```python
from build123d import *

# Parameters (mm, degrees)
F3_DEPTH  = 3
F4_W      = 23
F4_H      = 16
F5_DEPTH  = 11.6
F6_R      = 1.375
F7_DEPTH  = 2.75
F10_R     = 3.5
F11_DEPTH = 1.5
F12_R     = 2
F12_R_2   = 1
F13_DEPTH = 25


with BuildPart() as f1:
    # F0 (on Right) → F1 (revolve)
    with BuildSketch(Plane.YZ):
        Polygon((0, 2), (0, 0), (0.5, 0), (2, 2), align=None)
    revolve(axis=Axis((0, 0, 1), (0, 0, -1)))

    # F2 (on face) → F3 (join)
    with BuildSketch(Plane.XY.offset(2)):
        Polygon((2.020726, 3.5), (-2.020726, 3.5), (-4.041452, 0), (-2.020726, -3.5), (2.020726, -3.5), (4.041452, 0), align=None)
    extrude(amount=F3_DEPTH)

    # F4 (on face) → F5 (join)
    with BuildSketch(Plane.XY.offset(5)):
        with Locations((4.258548, 0)):
            Rectangle(F4_W, F4_H)
    extrude(amount=F5_DEPTH)

    # F6 (on face) → F7 (join)
    with BuildSketch(Plane.XY.offset(16.6)):
        Circle(F6_R)
    extrude(amount=F7_DEPTH)

    # F8 (on Front) → F9 (revolve)
    with BuildSketch(Plane.XZ):
        Polygon((0, 45.35), (0, 19.35), (1.375, 19.35), (11, 19.35), (11, 20.35), (6, 20.35), (5.89625, 21.85), (11, 21.85), (11, 22.85), (5.827083, 22.85), (5.723333, 24.35), (11, 24.35), (11, 25.35), (5.654167, 25.35), (5.550417, 26.85), (11, 26.85), (11, 27.85), (5.48125, 27.85), (5.3775, 29.35), (11, 29.35), (11, 30.35), (5.308333, 30.35), (5.204583, 31.85), (11, 31.85), (11, 32.85), (5.135417, 32.85), (5.031667, 34.35), (11, 34.35), (11, 35.35), (4.9625, 35.35), (4.85875, 36.85), (11, 36.85), (11, 37.85), (4.789583, 37.85), (4.685833, 39.35), (11, 39.35), (11, 40.35), (4.616667, 40.35), (4.512917, 41.85), (11, 41.85), (11, 42.85), (4.44375, 42.85), (4.34, 44.35), (11, 44.35), (11, 45.35), (4.270833, 45.35), (4.167083, 46.85), (8, 46.85), (8, 47.85), (4.097917, 47.85), (3.994167, 49.35), (8, 49.35), (8, 52.35), (6.25, 52.35), (6.25, 58.35), (8, 58.35), (8, 62.35), (0, 62.35), (0, 46.85), align=None)
    revolve(axis=Axis((0, 0, 40.529307), (0, 0, 1)))

    # F10 (on face) → F11 (join)
    with BuildSketch(Plane.XY.offset(62.35)):
        Circle(F10_R)
    extrude(amount=F11_DEPTH)

    # F12 (on face) → F13 (join)
    with BuildSketch(Plane.XY.offset(63.85)):
        Circle(F12_R)
        Circle(F12_R_2, mode=Mode.SUBTRACT)
    extrude(amount=F13_DEPTH)


solid = f1.part
```
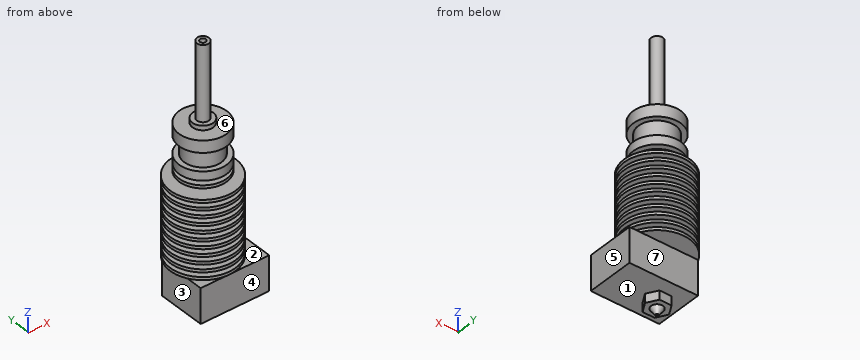
For this review, take the finished solid that the model builds, in its own axes (mm). Face numbers are marked on the shaded views. A direction names the side the tool comes from. Coordinates: 2 decimals unless noted, no trailing zeros. Order: outer loops, then holes, each group sorted by start corner. A loop starts at its lowest first (then second) coordinate and runs counter-clockwise, first axis right, second up. Notation, with made-up numbers: (80, 72) -> (98, 72) arc R16 cw to (98, 93) -> close; hole circle Ø6 at (7.25, -22). An arc over 180 degrees is marked (long way). Use CSV: the item, a comma, the result in double quotes. Start each with the question number.
Item 1: Wall thickness on probe 1 along Z at (x, y) = (2.25, 0.5); probe 2 along Y at (x, z) = (0, 76); probe 3 along Z at (x, y) = (3.25, -1.75): over which ranges is each line inside the solid? List them lowest first.
Item 2: For the marked faces 4, 5, 6 and 7, list the 3-axis set-ups (+Z, -Z, +X, -X, +Y, -Y) from which the entire face can be reached by the end or side of a thin tool; tool diameter is ignored.
Item 3: We need section B-B, the plane x = 12.5. Give the boundary of the cut face in (y, z), then the cut area to 3 significant figures.
Item 4: Draft analysis for pull direction Z (two halves, no side actions). For the marked faces 1, 2 and 3, state which applies: pulls with the +Z half, pulls with the -Z half, needs draft (parallel to the pull), parting line crosses it, or undercut.
Item 5: We need section A-A, the plane z = 18. Give the boundary of the cut face in (x, y) (3 decimals).
Item 6: Insertion check: pin 1 (5 mm diameter, centred on x = 13, y = 0.5, fed in from -Z); pin 2 (10 mm diameter, centred on y = -8.5, z = 25, fed in from +X); pin 3 (1.5 mm diameter, centred on x = 0.5, z = 78, fed in from -Y). Each pin has a flat end and moves straight along its axis. Give the tip position at first contact, or say it passes through.
Derived:
1,probe 1,"z = 2 to 16.6, 19.35 to 63.85"
1,probe 2,"y = -2 to -1, 1 to 2"
1,probe 3,"z = 5 to 16.6, 19.35 to 62.35"
2,face 4,"-Z, +X, -X, -Y"
2,face 5,"+Z, -Z, +X, +Y, -Y"
2,face 6,"+Z"
2,face 7,"-Z, +X, -X, +Y"
3,outline,"(-8, 5) -> (8, 5) -> (8, 16.6) -> (-8, 16.6) -> close"
3,area,"186 mm^2"
4,face 1,"pulls with the -Z half"
4,face 2,"undercut"
4,face 3,"needs draft"
5,outline,"circle Ø2.75 at (0, 0)"
6,pin 1,"stops at z = 5"
6,pin 2,"stops at x = 10.43"
6,pin 3,"stops at y = -2"
